Read the model definition and answer for the solid it produces. Units are mm, in the model's axes. Face numbers are marked on the shaded views. Give positions to 0.01 mm unless a question says otherwise; leave off trailing zeros. Write each loop counter-clockwise with the first axis right and the second up, starting at its lowest first coordinate (ties: lowest second). Pieces come first, ordered by that corner, then holes.
```python
from build123d import *

# Parameters (mm, degrees)
F0_R     = 231
F0_R_2   = 229
F1_DEPTH = 40
F2_W     = 30
F2_H     = 30
F3_DEPTH = 3
F4_R     = 4
F5_DEPTH = 25
F6_R     = 10
F8_COUNT = 4
F9_SIZE  = 2.99999


# Not quite as in the source:
# - a fillet or chamfer is up to 0.001 mm smaller than in the source, because OpenCascade refuses the exact size


with BuildPart() as f1:
    # F0 (on Top) → F1 (new body)
    with BuildSketch(Plane.XY):
        Circle(F0_R)
        Circle(F0_R_2, mode=Mode.SUBTRACT)
    extrude(amount=F1_DEPTH)

    # F2 (on face) → F3 (join)
    with BuildSketch(Plane(origin=(0, 0, 0), x_dir=(1, 0, 0), z_dir=(0, 0, -1))):
        with Locations((0, -245.5124725476)):
            Rectangle(F2_W, F2_H)
    extrude(amount=-F3_DEPTH)

    # F4 (on face) → F5 (cut)
    with BuildSketch(Plane(origin=(0, 0, 0), x_dir=(1, 0, 0), z_dir=(0, 0, -1))):
        with Locations((0, -245.5124725476)):
            Circle(F4_R)
    extrude(amount=-F5_DEPTH, mode=Mode.SUBTRACT)

    # F6
    f6_edges = [f1.edges().sort_by_distance(p)[0] for p in [
        (-15, 260.512473, 1.5),
        (15, 260.512473, 1.5),
    ]]
    fillet(f6_edges, radius=F6_R)

    # F8: F1 ×4 about axis
    f8_axis = Axis((0, 0, -51.1162020266), (0, 0, -1))


with BuildPart() as f1_1:
    add(f1.part)
    for i in range(1, F8_COUNT):
        add(f1.part.rotate(f8_axis, i * 360 / F8_COUNT))

    # F9 (size 3 in the source; OpenCascade refuses exactly that, so slightly less here)
    f9_edges = [f1_1.edges().sort_by_distance(p)[0] for p in [
        (-245.512473, -4, 3),
        (-4, 245.512473, 3),
        (245.512473, 4, 3),
        (4, -245.512473, 3),
    ]]
    chamfer(f9_edges, length=F9_SIZE)


solid = f1_1.part
```
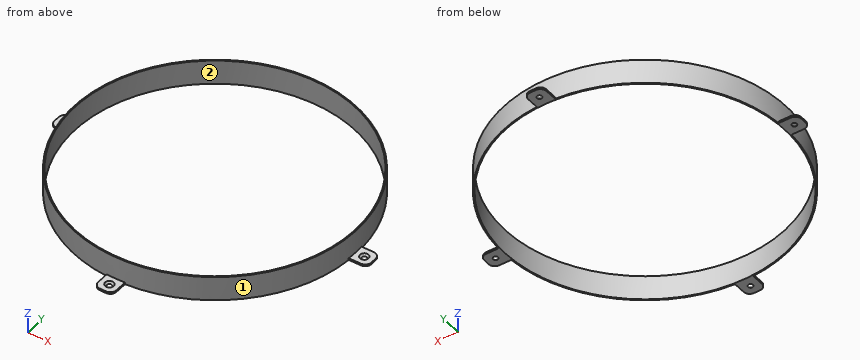
Item 1: Find the intervals of material crossed by line 1 along X through (y, z) = (0, 13); line 2 along Y through (x, z) = (108, 2.5); line 3 along X through (y, z) = (210, 33), in increasing order.
Result set:
line 1: x = -231 to -229, 229 to 231
line 2: y = -204.2 to -201.93, 201.93 to 204.2
line 3: x = -96.23 to -91.33, 91.33 to 96.23
Item 2: Determine the mould class of the marked faces 1 and 2 for opening direction X: pulls with the +X half, pulls with the -X half, needs draft (parallel to the pull), parting line crosses it, or undercut.
Result set:
face 1: parting line crosses it
face 2: undercut
Item 3: Section B-B (x = 161) is taken. Write down the section's boundary in (y, z).
Result set:
outline: (-165.65, 0) - (-162.85, 0) - (-162.85, 40) - (-165.65, 40) - close; (162.85, 0) - (165.65, 0) - (165.65, 40) - (162.85, 40) - close
Item 4: Section C-C (z = 27) is taken. Write down the section's boundary in (x, y).
Result set:
outline: circle Ø462 at (0, 0); hole circle Ø458 at (0, 0)
Item 5: Each of these flat-tipped pins is pushed along its axis until it touches: pin 1 Ø15 at (x, y) = (-251, -3.5) entering from +Z; pin 2 Ø3 at (y, z) = (-45, 34) entering from -X; pin 3 Ø5 at (x, z) = (13.5, 6.5) entering from -Y; pin 4 Ø5 at (x, y) = (0, -245.51) entering from -Z. Where does it stop, or does it pass through?
Result set:
pin 1: stops at z = 3
pin 2: stops at x = -226.87
pin 3: stops at y = -230.74
pin 4: passes through
